Geometry: final body of the model. Coordinates: model frame, mm. A direction names the side the tool comes from. Give positions to 0.01 mm unless a question says otherwise; leave off trailing zeros. Loops run counter-clockwise (first coordinate to the right, second up) from the corner with the lowest first, then second, coordinate; pieces in that order, holes last.
Autodesk Inventor part; units mm, degrees
ref_plane "YZ Plane" through (0, 0, 0) normal (1, 0, 0) x (0, 1, 0)
ref_plane "XZ Plane" through (0, 0, 0) normal (0, 1, 0) x (-1, 0, 0)
ref_plane "XY Plane" through (0, 0, 0) normal (0, 0, 1) x (1, 0, 0)
sketch "Boceto1" plane through (0, 0, 0) normal (0, 0, 1) x (1, 0, 0)
  arc A0 (6, 64.05) -> (4.45, 62.5) centre (6, 62.5) ccw
  arc A1 (4.45, 62.5) -> (6, 60.95) centre (6, 62.5) ccw
  arc A2 (6, 60.95) -> (7.55, 62.5) centre (6, 62.5) ccw
  arc A3 (7.55, 62.5) -> (6, 64.05) centre (6, 62.5) ccw
  arc A4 (55, 64.05) -> (53.45, 62.5) centre (55, 62.5) ccw
  arc A5 (53.45, 62.5) -> (55, 60.95) centre (55, 62.5) ccw
  arc A6 (55, 60.95) -> (56.55, 62.5) centre (55, 62.5) ccw
  arc A7 (56.55, 62.5) -> (55, 64.05) centre (55, 62.5) ccw
  arc A8 (104, 64.05) -> (102.45, 62.5) centre (104, 62.5) ccw
  arc A9 (102.45, 62.5) -> (104, 60.95) centre (104, 62.5) ccw
  arc A10 (104, 60.95) -> (105.55, 62.5) centre (104, 62.5) ccw
  arc A11 (105.55, 62.5) -> (104, 64.05) centre (104, 62.5) ccw
  arc A12 (6, 35.05) -> (4.45, 33.5) centre (6, 33.5) ccw
  arc A13 (4.45, 33.5) -> (6, 31.95) centre (6, 33.5) ccw
  arc A14 (6, 31.95) -> (7.55, 33.5) centre (6, 33.5) ccw
  arc A15 (7.55, 33.5) -> (6, 35.05) centre (6, 33.5) ccw
  arc A16 (55, 39.05) -> (53.45, 37.5) centre (55, 37.5) ccw
  arc A17 (53.45, 37.5) -> (55, 35.95) centre (55, 37.5) ccw
  arc A18 (55, 35.95) -> (56.55, 37.5) centre (55, 37.5) ccw
  arc A19 (56.55, 37.5) -> (55, 39.05) centre (55, 37.5) ccw
  arc A20 (104, 35.05) -> (102.45, 33.5) centre (104, 33.5) ccw
  arc A21 (102.45, 33.5) -> (104, 31.95) centre (104, 33.5) ccw
  arc A22 (104, 31.95) -> (105.55, 33.5) centre (104, 33.5) ccw
  arc A23 (105.55, 33.5) -> (104, 35.05) centre (104, 33.5) ccw
  arc A24 (6, 6.05) -> (4.45, 4.5) centre (6, 4.5) ccw
  arc A25 (4.45, 4.5) -> (6, 2.95) centre (6, 4.5) ccw
  arc A26 (6, 2.95) -> (7.55, 4.5) centre (6, 4.5) ccw
  arc A27 (7.55, 4.5) -> (6, 6.05) centre (6, 4.5) ccw
  arc A28 (104, 6.05) -> (102.45, 4.5) centre (104, 4.5) ccw
  arc A29 (102.45, 4.5) -> (104, 2.95) centre (104, 4.5) ccw
  arc A30 (104, 2.95) -> (105.55, 4.5) centre (104, 4.5) ccw
  arc A31 (105.55, 4.5) -> (104, 6.05) centre (104, 4.5) ccw
  arc A32 (40.5, 24.55) -> (38.95, 23) centre (40.5, 23) ccw
  arc A33 (38.95, 23) -> (40.5, 21.45) centre (40.5, 23) ccw
  arc A34 (40.5, 21.45) -> (42.05, 23) centre (40.5, 23) ccw
  arc A35 (42.05, 23) -> (40.5, 24.55) centre (40.5, 23) ccw
  arc A36 (40.5, 14.55) -> (38.95, 13) centre (40.5, 13) ccw
  arc A37 (38.95, 13) -> (40.5, 11.45) centre (40.5, 13) ccw
  arc A38 (40.5, 11.45) -> (42.05, 13) centre (40.5, 13) ccw
  arc A39 (42.05, 13) -> (40.5, 14.55) centre (40.5, 13) ccw
  arc A40 (20, 74.55) -> (18.45, 73) centre (20, 73) ccw
  arc A41 (18.45, 73) -> (20, 71.45) centre (20, 73) ccw
  arc A42 (20, 71.45) -> (21.55, 73) centre (20, 73) ccw
  arc A43 (21.55, 73) -> (20, 74.55) centre (20, 73) ccw
  arc A44 (90, 74.55) -> (88.45, 73) centre (90, 73) ccw
  arc A45 (88.45, 73) -> (90, 71.45) centre (90, 73) ccw
  arc A46 (90, 71.45) -> (91.55, 73) centre (90, 73) ccw
  arc A47 (91.55, 73) -> (90, 74.55) centre (90, 73) ccw
  line L0 (9.85, 75.35) -> (4.15, 75.35)
  line L1 (4.15, 75.35) -> (4.15, 70.65)
  line L2 (4.15, 70.65) -> (9.85, 70.65)
  line L3 (9.85, 70.65) -> (9.85, 75.35)
  line L4 (35.85, 70.65) -> (35.85, 75.35)
  line L5 (35.85, 75.35) -> (30.15, 75.35)
  line L6 (30.15, 75.35) -> (30.15, 70.65)
  line L7 (30.15, 70.65) -> (35.85, 70.65)
  line L8 (74.15, 70.65) -> (79.85, 70.65)
  line L9 (79.85, 70.65) -> (79.85, 75.35)
  line L10 (79.85, 75.35) -> (74.15, 75.35)
  line L11 (74.15, 75.35) -> (74.15, 70.65)
  line L12 (105.85, 70.65) -> (105.85, 75.35)
  line L13 (105.85, 75.35) -> (100.15, 75.35)
  line L14 (100.15, 75.35) -> (100.15, 70.65)
  line L15 (100.15, 70.65) -> (105.85, 70.65)
  line L16 (38.85, 44) -> (38.85, 56)
  line L17 (38.85, 56) -> (10.15, 56)
  line L18 (10.15, 56) -> (10.15, 44)
  line L19 (10.15, 44) -> (38.85, 44)
  line L20 (71.15, 44) -> (99.85, 44)
  line L21 (99.85, 44) -> (99.85, 56)
  line L22 (99.85, 56) -> (71.15, 56)
  line L23 (71.15, 56) -> (71.15, 44)
  line L24 (-0.2, -0.2) -> (110.2, -0.2)
  line L25 (110.2, -0.2) -> (110.2, 78.2)
  line L26 (110.2, 78.2) -> (69.8, 78.2)
  line L27 (69.8, 78.2) -> (69.8, 70.2)
  line L28 (69.8, 70.2) -> (40.2, 70.2)
  line L29 (40.2, 70.2) -> (40.2, 78.2)
  line L30 (40.2, 78.2) -> (-0.2, 78.2)
  line L31 (-0.2, 78.2) -> (-0.2, -0.2)
  arc A48 (28, 20.75) -> (25.25, 18) centre (28, 18) ccw
  arc A49 (25.25, 18) -> (28, 15.25) centre (28, 18) ccw
  arc A50 (28, 15.25) -> (30.75, 18) centre (28, 18) ccw
  arc A51 (30.75, 18) -> (28, 20.75) centre (28, 18) ccw
  arc A52 (53, 20.75) -> (50.25, 18) centre (53, 18) ccw
  arc A53 (50.25, 18) -> (53, 15.25) centre (53, 18) ccw
  arc A54 (53, 15.25) -> (55.75, 18) centre (53, 18) ccw
  arc A55 (55.75, 18) -> (53, 20.75) centre (53, 18) ccw
  point P0 (0, 0)
extrude "Extrusión1" add sketch "Boceto1" along normal blind 5
properties part number "carro x lado polea pieza1"
Item 1: Section query B-B on x = 15.5. Return loops of the section in (y, z).
Values follow:
outline: (-0.2, 0) - (44, 0) - (44, 5) - (-0.2, 5) - close; (56, 0) - (78.2, 0) - (78.2, 5) - (56, 5) - close
Item 2: Set-up query: faces 3 (the face through (40.2, 74, 2)), 4 (the face through (103, 75.35, 2)). Return all of +Z, -Z, +X, -X, +Y, -Y with unobstructed straight access to the full face (end or side cutting, diameter ignored); none if empty.
Values follow:
face 3: +Z, -Z, +Y
face 4: +Z, -Z
Item 3: Pin query (flat end, axial travel): pin 1 (3.5 mm diameter, centred on x = 104, y = 4.5, fed in from -Z). Return the tip coordinate at first contact, or that it passes through.
Values follow:
pin 1: stops at z = 0
Item 4: Section query C-C on y = 73. Give the number of separate pieces and of enclosed holes in the cut face, plus the area to 3 significant figures.
Values follow:
separate pieces: 8
enclosed holes: 0
area: 259 mm2
Item 5: Section query D-D on x = 104. Return loops of the section in (y, z).
Values follow:
outline: (-0.2, 0) - (2.95, 0) - (2.95, 5) - (-0.2, 5) - close; (6.05, 0) - (31.95, 0) - (31.95, 5) - (6.05, 5) - close; (35.05, 0) - (60.95, 0) - (60.95, 5) - (35.05, 5) - close; (64.05, 0) - (70.65, 0) - (70.65, 5) - (64.05, 5) - close; (75.35, 0) - (78.2, 0) - (78.2, 5) - (75.35, 5) - close
Item 6: Section query A-A on y = 47.5. Return loops of the section in (x, z), plus the area to 3 significant figures.
Values follow:
outline: (-0.2, 0) - (10.15, 0) - (10.15, 5) - (-0.2, 5) - close; (38.85, 0) - (71.15, 0) - (71.15, 5) - (38.85, 5) - close; (99.85, 0) - (110.2, 0) - (110.2, 5) - (99.85, 5) - close
area: 265 mm2
Item 7: Ray query, probe 1 along Y at (x, z) = (28, 1.5); probe 2 along Y at (x, z) = (79, 3.6); probe 3 along X at (y, z) = (4.5, 3.95). Return the intervals inside material, ascending.
Values follow:
probe 1: y = -0.2 to 15.25, 20.75 to 44, 56 to 78.2
probe 2: y = -0.2 to 44, 56 to 70.65, 75.35 to 78.2
probe 3: x = -0.2 to 4.45, 7.55 to 102.45, 105.55 to 110.2
Item 8: Draft query along X for faces 1 (the face through (54, -0.2, 2)), 2 (the face through (74.15, 73, 2)). Return one class per face: +X half, -X half, draft (parallel to the pull), parting line (faces both ways), or undercut.
Values follow:
face 1: draft
face 2: undercut
